```python
from build123d import *

# Parameters (mm, degrees)
F1_DEPTH = 10
F2_D     = 13
F3_D     = 13
F4_D     = 13


with BuildPart() as f1:
    # F0 (on Front) → F1 (new body)
    with BuildSketch(Plane.XZ):
        with BuildLine():
            ThreePointArc((14.88112472, 269.9518393504), (-15.11887528, 299.9518393504), (-45.11887528, 269.9518393504))
            Line((-45.11887528, 269.9518393504), (-45.11887528, -15.0481606496))
            ThreePointArc((-45.11887528, -15.0481606496), (-15.11887528, -45.0481606496), (14.88112472, -15.0481606496))
            Line((14.88112472, -15.0481606496), (14.88112472, 269.9518393504))
        make_face()
    extrude(amount=F1_DEPTH)

    # F2 (through all)
    with Locations(Plane(origin=(0, 0, 0), x_dir=(1, 0, 0), z_dir=(0, 1, 0))):
        with Locations((-15.11887528, -29.9518393504), (-15.11887528, 25.0481606496)):
            Hole(F2_D / 2)

    # F3 (through all)
    with Locations(Plane(origin=(0, 0, 0), x_dir=(1, 0, 0), z_dir=(0, 1, 0))):
        with Locations((-15.11887528, -279.9518393504)):
            Hole(F3_D / 2)

    # F4 (through all)
    with Locations(Plane(origin=(0, 0, 0), x_dir=(1, 0, 0), z_dir=(0, 1, 0))):
        with Locations((-25.11887528, -237.4518393504), (-5.11887528, -99.9518393504)):
            Hole(F4_D / 2)


solid = f1.part
```
The model under review builds one solid part; all positions refer to its coordinate system, in mm. Round coordinates to 2 decimals unless told otherwise and drop trailing zeros. Order: outer loops, then holes, each group sorted by start corner. A loop starts at its lowest first (then second) coordinate and runs counter-clockwise, first axis right, second up.
Item 1: Add section B-B, the plane y = -7. State the section outline as (x, z) points, and give its area (3 significant figures).
Working result:
outline: (-45.12, -15.05) arc R30 ccw to (14.88, -15.05) - (14.88, 269.95) arc R30 ccw to (-45.12, 269.95) - close; hole circle Ø13 at (-25.12, 237.45); hole circle Ø13 at (-15.12, -25.05); hole circle Ø13 at (-15.12, 29.95); hole circle Ø13 at (-15.12, 279.95); hole circle Ø13 at (-5.12, 99.95)
area: 19,300 mm2
Item 2: Draft analysis for pull direction Z (two halves, no side actions). For faces 1 (the cylindrical face through (-23.71, -5.07, 243.797)), 2 (the cylindrical face through (-14.459, -4.93, 299.945)), 3 (the cylindrical face through (-15.78, -4.93, -45.04)), state which applies: released by +Z, released by -Z, zero draft, split by the parting line, or undercut.
Working result:
face 1: undercut
face 2: released by +Z
face 3: released by -Z
Item 3: To check wall thickness, follow probe 1 along Z at (x, y) = (-20, -8); probe 2 along Z at (x, y) = (-18, -2.5); probe 3 along Z at (x, y) = (-22, -1.75). State the ranges of each line that lie inside material, in increasing order.
Working result:
probe 1: z = -44.65 to -29.34, -20.76 to 25.66, 34.24 to 233.45, 241.46 to 275.66, 284.24 to 299.55
probe 2: z = -44.91 to -30.87, -19.22 to 24.13, 35.78 to 274.13, 285.78 to 299.81
probe 3: z = -44.25 to 231.75, 243.15 to 299.15
Item 4: Add section A-A, the plane z = 97. State the section outline as (x, y) points, and give its area (3 significant figures).
Working result:
outline: (-45.12, -10) - (-10.91, -10) - (-10.91, 0) - (-45.12, 0) - close; (0.67, -10) - (14.88, -10) - (14.88, 0) - (0.67, 0) - close
area: 484 mm2
Item 5: For pin 1 (8 mm diameter, centred on x = -15.12, z = -25.05, fed in from +Y); pin 2 (5 mm diameter, centred on x = -5.5, y = -2, fed in from -Z); pin 3 (1 mm diameter, centred on x = -2, y = -6.5, fed in from +Z), all flat-tipped, find the tip position at first contact; note any pin that passes through.
Working result:
pin 1: passes through
pin 2: stops at z = -44.19
pin 3: stops at z = 297.17
Item 6: Add section C-C, the plane x = 8. State the section outline as (y, z) points.
Working result:
outline: (-10, -34.17) - (0, -34.17) - (0, 289.07) - (-10, 289.07) - close
